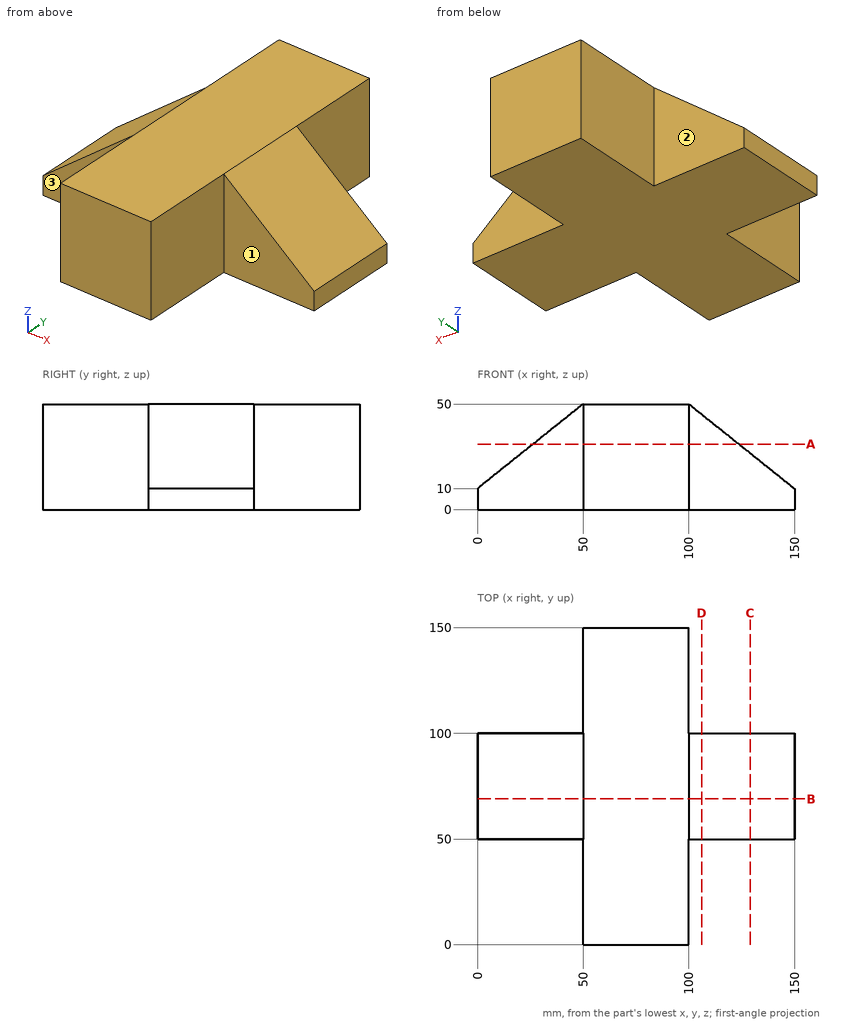
Part print with two shaded views. Sizes in mm from the minimum x, y, z corner. A direction names the side the tool comes from. Round coordinates to 2 decimals unless told otherwise and drop trailing zeros. Loops run counter-clockwise (first coordinate to the right, second up) from the corner with the lowest first, then second, coordinate; pieces in that order, holes last. Notation, with made-up numbers: M 37.25,70.25 L 43.25,70.25 A13 cw 43.25,91.25 Z; hole C 73.5,-18.5 d4. An arc over 180 degrees is marked long. Put each result on its own line as item: value. Start each with the question number.
Item 1: Cut at C-C (x = 129). List the corners of the cut face in (y, z).
Item 2: Cut at D-D (x = 106). List the corners of the cut face in (y, z).
Item 3: Drill centre lines: line 1 along X through (y, z) = (122, 5.5); line 2 along Z through (x, y) = (33.5, 64.5). Where is each one in solid material? Low to high.
Item 4: Cut at B-B (y = 69). List the corners of the cut face in (x, z), then the cut area to 3 significant figures.
Item 5: Drop flat-ended pins along their axis: P1, Ø8, axis at y = 88.5, z = 37, coming from the +X side; P2, Ø2, axis at x = 33.5, y = 102, coming from the +Z side; P3, Ø25, axis at x = 131.5, z = 25, coming from the +Y side; P4, Ø12, axis at y = 73, z = 25.5, coming from the -X side (3 decimals). Give the stop position or say it passes through.
Item 6: Cut at A-A (z = 31). List the corners of the cut face in (x, y), then the cut area to 4 significant figures.
Item 7: 3-axis set-ups, long thin cutter, end or side, ignore diameter. For the marked faces 1, 2 and 3: which of +Z, -Z, +X, -X, +Y, -Y reach the whole face in a straight line?
Answer block:
1. outline: M 50,0 L 100,0 L 100,26.8 L 50,26.8 Z
2. outline: M 50,0 L 100,0 L 100,45.2 L 50,45.2 Z
3. line 1: 50 to 100
3. line 2: 0 to 36.8
4. outline: M 0,0 L 150,0 L 150,10 L 100,50 L 50,50 L 0,10 Z
4. area: 5,500 mm2
5. P1: x = 121.25
5. P2: through
5. P3: y = 100
5. P4: x = 11.875
6. outline: M 26.25,50 L 50,50 L 50,0 L 100,0 L 100,50 L 123.75,50 L 123.75,100 L 100,100 L 100,150 L 50,150 L 50,100 L 26.25,100 Z
6. area: 9,875 mm2
7. face 1: +Z, -Z, +X, -Y
7. face 2: +Z, -Z, -X, +Y
7. face 3: +Z, -Z, -X, -Y
